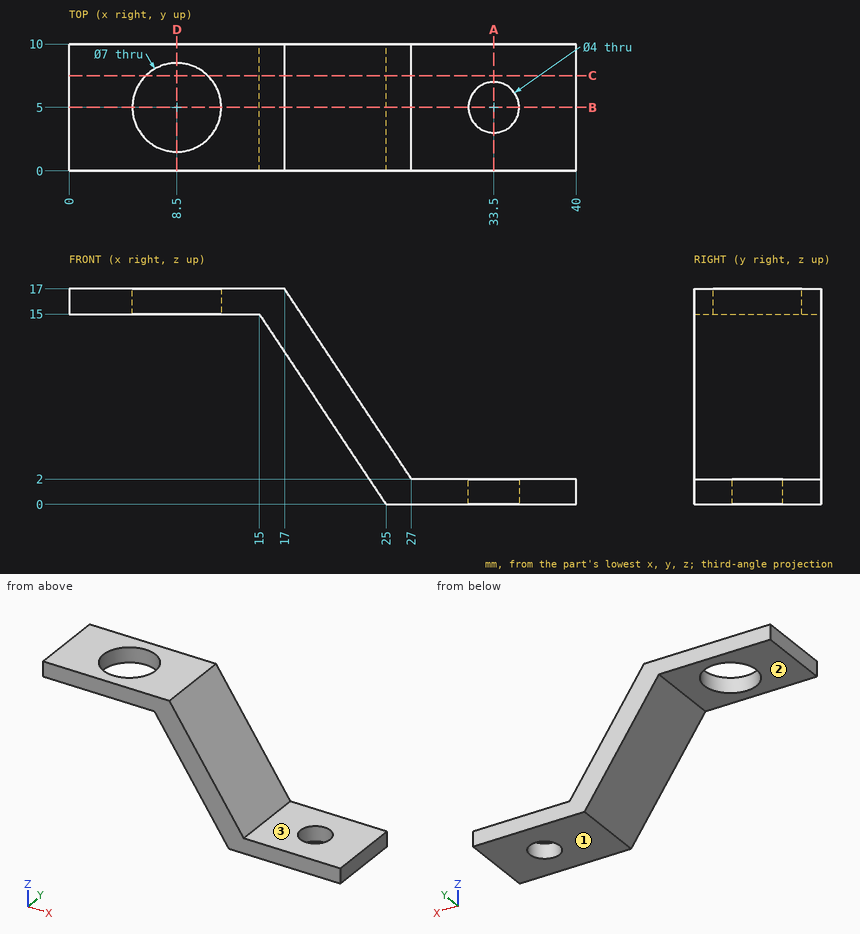
Input: dimensioned drawing with shaded views. Units: mm. Origin: part minimum x, y, z. A direction names the side the tool comes from. Round coordinates to 2 decimals unless told otherwise and drop trailing zeros. Loops run counter-clockwise (first coordinate to the right, second up) from the corner with the lowest first, then second, coordinate; pieces in that order, holes last. Notation, with made-up numbers: (4, -32) -> (15, -32) arc R16 ccw to (15, -3) -> close; hole circle Ø6 at (74, -38.5). An arc over 180 degrees is marked (long way). Use one line per item in the form item = value. Start each with the question number.
1) First-contact query: P1, Ø3, axis at y = 1, z = 6, coming from the +X side; P2, Ø3, axis at y = 6.5, z = 5.5, coming from the +X side; P3, Ø4, axis at x = 28.5, y = 5.5, coming from the +Z side. Flat tips, straight axial feed; report the tip coordinate or a pass-through.
2) Line query: L1, parallel to Y at x = 8.5, z = 15.7; L2, parallel to Z at x = 29, y = 3.75; L3, parallel to Z at x = 14, y = 4.75. Output: solid intervals per line, ascending.
3) Section A-A on x = 33.5. Output: boundary loops of the cut face in (y, z), then the cut area to 3 significant figures.
4) Section B-B on y = 5. Output: boundary loops of the cut face in (x, z).
5) Access query for the marked faces 1, 2 and 3. Directions: +Z, -Z, +X, -X, +Y, -Y. A direction counts if a zero-diameter tool reaches every point of the face in a straight line with its end or side. Return the directions, or none.
6) Section D-D on x = 8.5. Output: boundary loops of the cut face in (y, z).
7) Section C-C on y = 7.5. Output: boundary loops of the cut face in (x, z), then the cut area to 3 significant figures.
Response:
q1.P1 = 25.33
q1.P2 = 25.67
q1.P3 = 2.75
q2.L1 = 0 to 1.5, 8.5 to 10
q2.L2 = 0 to 2
q2.L3 = 15 to 17
q3.outline = (0, 0) -> (3, 0) -> (3, 2) -> (0, 2) -> close; (7, 0) -> (10, 0) -> (10, 2) -> (7, 2) -> close
q3.area = 12.0 mm^2
q4.outline = (0, 15) -> (5, 15) -> (5, 17) -> (0, 17) -> close; (12, 15) -> (15, 15) -> (25, 0) -> (31.5, 0) -> (31.5, 2) -> (27, 2) -> (17, 17) -> (12, 17) -> close; (35.5, 0) -> (40, 0) -> (40, 2) -> (35.5, 2) -> close
q5.face_1 = -Z, +X, -X, +Y, -Y
q5.face_2 = -Z, -X, +Y, -Y
q5.face_3 = +Z, +X, +Y, -Y
q6.outline = (0, 15) -> (1.5, 15) -> (1.5, 17) -> (0, 17) -> close; (8.5, 15) -> (10, 15) -> (10, 17) -> (8.5, 17) -> close
q7.outline = (0, 15) -> (6.05, 15) -> (6.05, 17) -> (0, 17) -> close; (10.95, 15) -> (15, 15) -> (25, 0) -> (40, 0) -> (40, 2) -> (27, 2) -> (17, 17) -> (10.95, 17) -> close
q7.area = 100 mm^2
